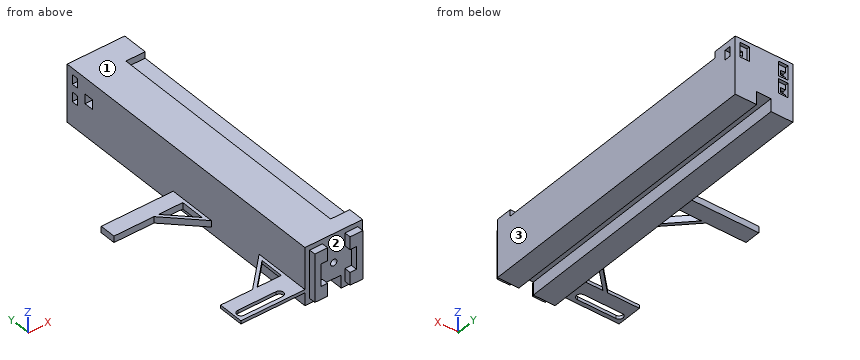
```python
from build123d import *

# Parameters (mm, degrees)
SKETCH1_W           = 36
SKETCH1_H           = 36
BOSS_EXTRUDE1_DEPTH = 186.9
BOSS_EXTRUDE2_DEPTH = 4
SKETCH3_R           = 2
CUT_EXTRUDE1_DEPTH  = 5
SKETCH4_W           = 9
SKETCH4_H           = 186.9
CUT_EXTRUDE2_DEPTH  = 8
SKETCH5_W           = 6
SKETCH5_H           = 4
CUT_EXTRUDE3_DEPTH  = 9
SKETCH6_W           = 3
SKETCH6_H           = 3
CUT_EXTRUDE4_DEPTH  = 10
SKETCH7_W           = 2
SKETCH7_H           = 16
BOSS_EXTRUDE3_DEPTH = 40
CUT_EXTRUDE5_REACH  = 12
SKETCH9_W           = 4
SKETCH9_H           = 10
BOSS_EXTRUDE4_DEPTH = 45
CHAMFER1_SIZE       = 20
CUT_EXTRUDE6_DEPTH  = 27
SKETCH11_W          = 6
SKETCH11_H          = 4
SKETCH11_H_2        = 6
CUT_EXTRUDE7_DEPTH  = 9
SKETCH12_W          = 3
SKETCH12_H          = 3
CUT_EXTRUDE8_DEPTH  = 10
SKETCH13_W          = 12
SKETCH13_H          = 160.9
CUT_EXTRUDE9_DEPTH  = 4
SKETCH14_W          = 6
SKETCH14_H          = 9
CUT_EXTRUDE10_DEPTH = 2


with BuildPart() as part:
    # Sketch1 → Boss-Extrude1 (new body)
    with BuildSketch(Plane(origin=(0, 0, 0), x_dir=(1, 0, 0), z_dir=(0, 1, 0))):
        with Locations((18, 18)):
            Rectangle(SKETCH1_W, SKETCH1_H)
    extrude(amount=BOSS_EXTRUDE1_DEPTH)

    # Sketch2 → Boss-Extrude2 (add)
    with BuildSketch(Plane.XZ):
        Polygon((3, -3), (7, -3), (11, -3), (11, -11), (7, -11), (7, -25), (11, -25), (11, -33), (7, -33), (3, -33), align=None)
        Polygon((29, -3), (33, -3), (33, -33), (29, -33), (25, -33), (25, -25), (29, -25), (29, -11), (25, -11), (25, -3), align=None)
    extrude(amount=BOSS_EXTRUDE2_DEPTH)

    # Sketch3 → Cut-Extrude1 (cut)
    with BuildSketch(Plane.XZ):
        with Locations((18, -18)):
            Circle(SKETCH3_R)
    extrude(amount=-CUT_EXTRUDE1_DEPTH, mode=Mode.SUBTRACT)

    # Sketch4 → Cut-Extrude2 (cut)
    with BuildSketch(Plane.XY.offset(-36)):
        with Locations((18.12, 93.45)):
            Rectangle(SKETCH4_W, SKETCH4_H)
    extrude(amount=CUT_EXTRUDE2_DEPTH, mode=Mode.SUBTRACT)

    # Sketch5 → Cut-Extrude3 (cut)
    with BuildSketch(Plane(origin=(36, 0, 0), x_dir=(0, 0, -1), z_dir=(1, 0, 0))):
        with Locations((7, 180.9)):
            Rectangle(SKETCH5_W, SKETCH5_H)
    extrude(amount=-CUT_EXTRUDE3_DEPTH, mode=Mode.SUBTRACT)

    # Sketch6 → Cut-Extrude4 (cut)
    with BuildSketch(Plane(origin=(0, 186.9, 0), x_dir=(1, 0, 0), z_dir=(0, 1, 0))):
        with Locations((31.5, 7)):
            Rectangle(SKETCH6_W, SKETCH6_H)
    extrude(amount=-CUT_EXTRUDE4_DEPTH, mode=Mode.SUBTRACT)

    # Sketch7 → Boss-Extrude3 (add)
    with BuildSketch(Plane.ZY):
        with Locations((-27, 8)):
            Rectangle(SKETCH7_W, SKETCH7_H)
    extrude(amount=BOSS_EXTRUDE3_DEPTH)

    # Sketch8 → Cut-Extrude5 (cut, up to next)
    with BuildSketch(Plane.XY.offset(-26), mode=Mode.PRIVATE) as cut_extrude5_sk1:
        with BuildLine():
            Line((-36, 7.5), (-12, 7.5))
            ThreePointArc((-12, 7.5), (-9.5, 5), (-12, 2.5))
            Line((-12, 2.5), (-36, 2.5))
            ThreePointArc((-36, 2.5), (-38.5, 5), (-36, 7.5))
        make_face()
    cut_extrude5_tool1 = extrude(cut_extrude5_sk1.sketch, amount=-CUT_EXTRUDE5_REACH, mode=Mode.PRIVATE) & part.part
    add(cut_extrude5_tool1.solids().sort_by_distance((-24, 5, -26))[0], mode=Mode.SUBTRACT)

    # Sketch9 → Boss-Extrude4 (add)
    with BuildSketch(Plane.ZY):
        with Locations((-30, 98.5)):
            Rectangle(SKETCH9_W, SKETCH9_H)
    extrude(amount=BOSS_EXTRUDE4_DEPTH)

    # Chamfer1
    chamfer1_edges = [part.edges().sort_by_distance(p)[0] for p in [
        (0, 16, -27),
        (0, 93.5, -30),
    ]]
    chamfer(chamfer1_edges, length=CHAMFER1_SIZE)

    # Sketch10 → Cut-Extrude6 (cut)
    with BuildSketch(Plane.XY.offset(-26)):
        Polygon((-17.171572875, 93.5), (-2, 78.328427125), (-2, 93.5), align=None)
        Polygon((-17.171572875, 16), (-2, 31.171572875), (-2, 16), align=None)
    extrude(amount=-CUT_EXTRUDE6_DEPTH, mode=Mode.SUBTRACT)

    # Sketch11 → Cut-Extrude7 (cut)
    with BuildSketch(Plane.ZY):
        with Locations((-7, 180.9)):
            Rectangle(SKETCH11_W, SKETCH11_H)
        with Locations((-17.8, 180.9)):
            Rectangle(SKETCH11_W, SKETCH11_H)
        with Locations((-13, 169.9)):
            Rectangle(SKETCH11_W, SKETCH11_H_2)
    extrude(amount=-CUT_EXTRUDE7_DEPTH, mode=Mode.SUBTRACT)

    # Sketch12 → Cut-Extrude8 (cut)
    with BuildSketch(Plane(origin=(0, 186.9, 0), x_dir=(1, 0, 0), z_dir=(0, 1, 0))):
        with Locations((4.5, 7)):
            Rectangle(SKETCH12_W, SKETCH12_H)
        with Locations((4.5, 17.8)):
            Rectangle(SKETCH12_W, SKETCH12_H)
    extrude(amount=-CUT_EXTRUDE8_DEPTH, mode=Mode.SUBTRACT)

    # Sketch13 → Cut-Extrude9 (cut)
    with BuildSketch(Plane.XY):
        with Locations((30, 90.45)):
            Rectangle(SKETCH13_W, SKETCH13_H)
    extrude(amount=-CUT_EXTRUDE9_DEPTH, mode=Mode.SUBTRACT)

    # Sketch14 → Cut-Extrude10 (cut)
    with BuildSketch(Plane(origin=(0, 186.9, 0), x_dir=(1, 0, 0), z_dir=(0, 1, 0))):
        with Locations((30, 7)):
            Rectangle(SKETCH14_W, SKETCH14_H)
        with Locations((6, 17.8)):
            Rectangle(SKETCH14_W, SKETCH14_H)
        with Locations((6, 7)):
            Rectangle(SKETCH14_W, SKETCH14_H)
    extrude(amount=-CUT_EXTRUDE10_DEPTH, mode=Mode.SUBTRACT)


solid = part.part
```
CAD build for the part. Positions are in the model's coordinates, mm. Face numbers are marked on the shaded views. Give positions to 0.01 mm unless a question says otherwise; leave off trailing zeros. Order: outer loops, then holes, each group sorted by start corner. A loop starts at its lowest first (then second) coordinate and runs counter-clockwise, first axis right, second up.
(1) Saw through at A-A, the plane y = 44. Give the cut face in (x, z), then the cut area to 3 significant figures.
(2) Drill centre lines: L1, parallel to Z at x = 18, y = 1.55; L2, parallel to X at y = 104.5, z = -31.5; L3, parallel to Z at x = -14, y = 103. Where is each one in solid material? Low to high.
(3) Mould opens along X. For the marked faces 1, 2 and 3 say: released by +X, released by -X, zero draft, split by the parting line, or undercut.
(4) Saw through at B-B, the plane x = 18. Give the cut face in (y, z).
(5) Flat gauge pins, fed straight in: pin 1 (10 mm diameter, centred on y = 115.5, z = -20, fed in from -X); pin 2 (2 mm diameter, centred on x = 4, y = 180.5, fed in from +Z); pin 3 (1 mm diameter, centred on x = -29.5, z = -27, fed in from +Y); pin 4 (3 mm diameter, centred on x = 5.5, y = -2.5, fed in from +Z). Where does each tip first touch, or does it go through?
Results found:
1. outline: (0, -36) - (13.62, -36) - (13.62, -28) - (22.62, -28) - (22.62, -36) - (36, -36) - (36, -4) - (24, -4) - (24, 0) - (0, 0) - close
1. area: 1,180 mm2
2. L1: z = -28 to -20, -16 to 0
2. L2: x = 0 to 13.62, 22.62 to 36
2. L3: z = -32 to -28
3. face 1: zero draft
3. face 2: undercut
3. face 3: released by +X
4. outline: (0, -28) - (186.9, -28) - (186.9, 0) - (0, 0) - (0, -16) - (5, -16) - (5, -20) - (0, -20) - close
5. pin 1: stops at x = 0
5. pin 2: stops at z = 0
5. pin 3: stops at y = 16
5. pin 4: stops at z = -3
